Build history of the part. All positions in model axes, mm. Round coordinates to 2 decimals unless told otherwise and drop trailing zeros. Write each loop counter-clockwise with the first axis right and the second up, starting at its lowest first coordinate (ties: lowest second). Pieces come first, ordered by that corner, then holes. Notation, with made-up numbers: (-29, 79.25) - (19, 79.25) arc R7 cw to (19, 91.25) - close; hole circle Ø1 at (19, -14). An arc over 180 degrees is marked (long way). Write each question's results on one line, items separated by ' | '.
from build123d import *

# Parameters (mm, degrees)
F1_DEPTH = 540
F2_W     = 31
F2_H     = 25
F3_DEPTH = 15
F4_W     = 31
F4_H     = 25
F5_DEPTH = 15
F6_R     = 2
F7_DEPTH = 10.001
F8_R     = 3.5
F9_DEPTH = 4
F10_R    = 1
F11_R    = 1


# Not quite as in the source:
# - a pattern or mirror of a feature is missing from the dataset's text; its kind, count and spacing are read off the source's solid


with BuildPart() as f1:
    # F0 (on Right) → F1 (new body, symmetric)
    with BuildSketch(Plane.YZ):
        Polygon((18.5, 12.5), (-18.5, 12.5), (-18.5, 2.5), (-15.5, 2.5), (-15.5, -22.5), (-10.5, -22.5), (-10.5, 2.5), (0, 2.5), (10.5, 2.5), (10.5, -22.5), (15.5, -22.5), (15.5, 2.5), (18.5, 2.5), align=None)
    extrude(amount=F1_DEPTH, both=True)

    # F2 (on face) → F3 (cut)
    with BuildSketch(Plane(origin=(-540, 0, 0), x_dir=(0, -1, 0), z_dir=(-1, 0, 0))):
        with Locations((0, -10)):
            Rectangle(F2_W, F2_H)
    extrude(amount=-F3_DEPTH, mode=Mode.SUBTRACT)

    # F4 (on face) → F5 (cut)
    with BuildSketch(Plane.YZ.offset(540)):
        with Locations((0, -10)):
            Rectangle(F4_W, F4_H)
    extrude(amount=-F5_DEPTH, mode=Mode.SUBTRACT)

    # F6 (on face) → F7 (cut, through all)
    with BuildSketch(Plane(origin=(0, 0, 2.5), x_dir=(1, 0, 0), z_dir=(0, 0, -1))):
        with Locations((-532.5, 9)):
            Circle(F6_R)
        with Locations((-532.5, -9)):
            Circle(F6_R)
    f7 = extrude(amount=-F7_DEPTH, mode=Mode.SUBTRACT)

    # F7_copies: F7 across plane
    add(f7.mirror(Plane(origin=(0, 0, 0), x_dir=(0, 0, 1), z_dir=(1, 0, 0))), mode=Mode.SUBTRACT)

    # F8 (on face) → F9 (cut)
    with BuildSketch(Plane.XY.offset(12.5)):
        with Locations((-532.5, -9)):
            Circle(F8_R)
        with Locations((-532.5, 9)):
            Circle(F8_R)
    f9 = extrude(amount=-F9_DEPTH, mode=Mode.SUBTRACT)

    # F9_copies: F9 across plane
    add(f9.mirror(Plane(origin=(0, 0, 0), x_dir=(0, 0, 1), z_dir=(1, 0, 0))), mode=Mode.SUBTRACT)

    # F10
    f10_edges = [f1.edges().sort_by_distance(p)[0] for p in [
        (540, 18.5, 7.5),
        (540, -18.5, 7.5),
        (525, 13, -22.5),
        (525, -13, -22.5),
        (-540, -18.5, 7.5),
        (-525, -13, -22.5),
        (-525, 13, -22.5),
        (-540, 18.5, 7.5),
    ]]
    fillet(f10_edges, radius=F10_R)

    # F11
    f11_edges = [f1.edges().sort_by_distance(p)[0] for p in [
        (-525, -10.5, -9.5),
        (-525, -15.5, -9.5),
        (-525, 15.5, -9.5),
        (-525, 10.5, -9.5),
        (-525, 13, -21.5),
        (-525, 13, 2.5),
        (-540, 0, 2.5),
        (-540, 0, 12.5),
        (0, -15.5, 2.5),
        (-539.707107, 18.207107, 12.5),
        (-539.707107, -18.207107, 12.5),
        (0, 18.5, 12.5),
        (0, -18.5, 12.5),
        (539.707107, 18.207107, 12.5),
        (539.707107, -18.207107, 12.5),
        (540, 0, 12.5),
        (-539.707107, 18.207107, 2.5),
        (-539.707107, -18.207107, 2.5),
        (0, 18.5, 2.5),
        (0, -18.5, 2.5),
        (539.707107, 18.207107, 2.5),
        (539.707107, -18.207107, 2.5),
        (540, 0, 2.5),
        (-525, -13, 2.5),
        (525, -13, 2.5),
        (0, -10.5, 2.5),
        (0, 10.5, 2.5),
        (525, 13, 2.5),
        (0, 15.5, 2.5),
        (525, -15.5, -9.5),
        (524.707107, -15.5, -22.207107),
        (0, -15.5, -22.5),
        (-524.707107, -15.5, -22.207107),
        (525, -10.5, -9.5),
        (0, -10.5, -22.5),
        (-524.707107, -10.5, -22.207107),
        (524.707107, -10.5, -22.207107),
        (525, 10.5, -9.5),
        (524.707107, 10.5, -22.207107),
        (0, 10.5, -22.5),
        (-524.707107, 10.5, -22.207107),
        (525, 15.5, -9.5),
        (0, 15.5, -22.5),
        (-524.707107, 15.5, -22.207107),
        (524.707107, 15.5, -22.207107),
    ]]
    fillet(f11_edges, radius=F11_R)


solid = f1.part
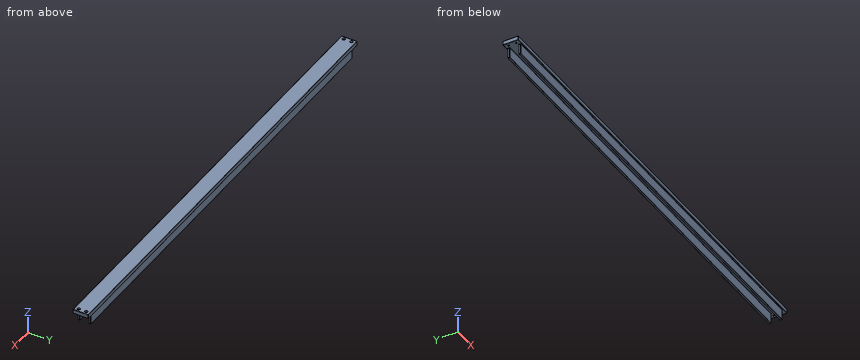
(1) Slice it at B-B, the plane z = -4. Write the cut outline in (x, y).
Worked answers:
outline: (-525, -14.5) arc R1 ccw to (-524, -15.5) - (524, -15.5) arc R1 ccw to (525, -14.5) - (525, -11.5) arc R1 ccw to (524, -10.5) - (-524, -10.5) arc R1 ccw to (-525, -11.5) - close; (-525, 11.5) arc R1 ccw to (-524, 10.5) - (524, 10.5) arc R1 ccw to (525, 11.5) - (525, 14.5) arc R1 ccw to (524, 15.5) - (-524, 15.5) arc R1 ccw to (-525, 14.5) - close
(2) Flat gauge pins, fed straight in: pin 1 Ø2.5 at (y, z) = (-13, -8.5) entering from +X; pin 2 Ø1.5 at (x, z) = (-116.5, -11) entering from -Y; pin 3 Ø1.5 at (y, z) = (13, -8) entering from -X; pin 4 Ø3.5 at (x, y) = (532.5, -9) entering from +Z. Where does each tip first touch, or does it go through?
Worked answers:
pin 1: stops at x = 525 | pin 2: stops at y = -15.5 | pin 3: stops at x = -525 | pin 4: passes through
(3) Drill centre lines: probe 1 along Y at (x, z) = (-532.5, 10.9); probe 2 along Y at (x, z) = (-532, 5); probe 3 along X at (y, z) = (-9, 6). Where is each one in solid material? Low to high. Write a range as [from, to].
Worked answers:
probe 1: y = [-18.5, -12.5], [-5.5, 5.5], [12.5, 18.5] | probe 2: y = [-18.5, -10.94], [-7.06, 7.06], [10.94, 18.5] | probe 3: x = [-540, -534.5], [-530.5, 530.5], [534.5, 540]
(4) Slice it at A-A, the plane x = 126. Write the cut outline in (y, z).
Worked answers:
outline: (-18.5, 3.5) arc R1 ccw to (-17.5, 2.5) - (-16.5, 2.5) arc R1 cw to (-15.5, 1.5) - (-15.5, -21.5) arc R1 ccw to (-14.5, -22.5) - (-11.5, -22.5) arc R1 ccw to (-10.5, -21.5) - (-10.5, 1.5) arc R1 cw to (-9.5, 2.5) - (9.5, 2.5) arc R1 cw to (10.5, 1.5) - (10.5, -21.5) arc R1 ccw to (11.5, -22.5) - (14.5, -22.5) arc R1 ccw to (15.5, -21.5) - (15.5, 1.5) arc R1 cw to (16.5, 2.5) - (17.5, 2.5) arc R1 ccw to (18.5, 3.5) - (18.5, 11.5) arc R1 ccw to (17.5, 12.5) - (-17.5, 12.5) arc R1 ccw to (-18.5, 11.5) - close
